CAD build for the part. Positions are in the model's coordinates, mm. Face numbers are marked on the shaded views. A direction names the side the tool comes from. Coordinates: 2 decimals unless noted, no trailing zeros. Loops run counter-clockwise (first coordinate to the right, second up) from the corner with the lowest first, then second, coordinate; pieces in that order, holes last. Notation, with made-up numbers: (-9, 17) - (0, 17) arc R28 cw to (0, 39) - close; hole circle Ø9 at (23, 7). An arc over 180 degrees is marked (long way). Put each result on its own line as item: value.
```python
from build123d import *

# Parameters (mm, degrees)
SKETCH1_R           = 60
BOSS_EXTRUDE1_DEPTH = 20
BOSS_EXTRUDE2_DEPTH = 10
SKETCH6_R           = 20.05
CUT_EXTRUDE1_DEPTH  = 92.787798753
SKETCH8_R           = 6.5
CUT_EXTRUDE3_DEPTH  = 10
SKETCH9_R           = 2.000000002
CUT_EXTRUDE4_DEPTH  = 20
SKETCH10_R          = 3.999999996
CUT_EXTRUDE5_DEPTH  = 4


with BuildPart() as part:
    # Sketch1 → Boss-Extrude1 (new body)
    with BuildSketch(Plane(origin=(0, 0, 0), x_dir=(1, 0, 0), z_dir=(0, 1, 0))):
        with Locations(Location((0, 0, 0), (0, 0, 270))):
            Circle(SKETCH1_R)
    extrude(amount=BOSS_EXTRUDE1_DEPTH)

    # Sketch2 → Boss-Extrude2 (add)
    with BuildSketch(Plane.XY.offset(45)):
        with BuildLine():
            Line((-37.344891303, 20), (-37.344891303, 30))
            ThreePointArc((-37.344891303, 30), (-12.344891303, 55), (12.655108697, 30))
            Line((12.655108697, 30), (12.655108697, 20))
            Line((12.655108697, 20), (-37.344891303, 20))
        make_face()
    extrude(amount=-BOSS_EXTRUDE2_DEPTH)

    # Sketch6 → Cut-Extrude1 (cut, through all)
    with BuildSketch(Plane(origin=(0, 20, 0), x_dir=(1, 0, 0), z_dir=(0, 1, 0))):
        with Locations(Location((0, 0, 0), (0, 0, 270))):
            Circle(SKETCH6_R)
    extrude(amount=-CUT_EXTRUDE1_DEPTH, mode=Mode.SUBTRACT)

    # Sketch8 → Cut-Extrude3 (cut)
    with BuildSketch(Plane.XY.offset(45)):
        with Locations((-12.344891303, 40)):
            Circle(SKETCH8_R)
    extrude(amount=-CUT_EXTRUDE3_DEPTH, mode=Mode.SUBTRACT)

    # Sketch9 → Cut-Extrude4 (cut)
    with BuildSketch(Plane(origin=(0, 20, 0), x_dir=(1, 0, 0), z_dir=(0, 1, 0))):
        with Locations(Location((45.655108698, 23.978394329, 0), (0, 0, 270))):
            Circle(SKETCH9_R)
        with Locations(Location((-32.344891302, 23.978394329, 0), (0, 0, 270))):
            Circle(SKETCH9_R)
    extrude(amount=-CUT_EXTRUDE4_DEPTH, mode=Mode.SUBTRACT)

    # Sketch10 → Cut-Extrude5 (cut)
    with BuildSketch(Plane.XZ):
        with Locations(Location((45.655108698, -23.978394329, 0), (0, 0, 270))):
            Circle(SKETCH10_R)
        with Locations(Location((-32.344891302, -23.978394329, 0), (0, 0, 270))):
            Circle(SKETCH10_R)
    extrude(amount=-CUT_EXTRUDE5_DEPTH, mode=Mode.SUBTRACT)


solid = part.part
```
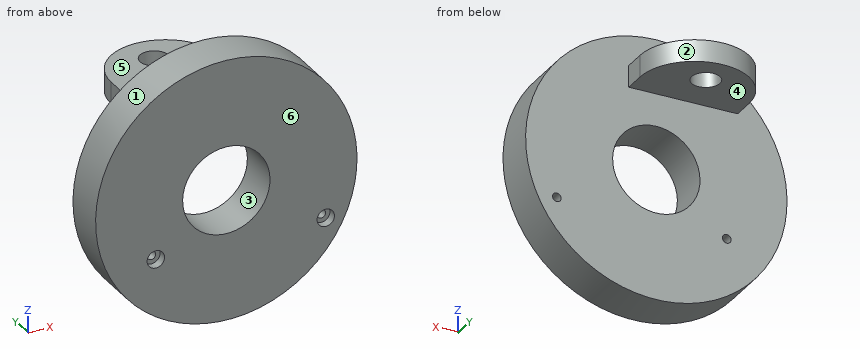
Q1. Tool access for the marked faces 4, 5 and 6: list every direction of +Z, -Z, +X, -X, +Y, -Y with a clear straight run to the whole face (end or side of a thin tool).
Determined:
face 4: -Z, +X, -X, +Y
face 5: +Z, +X, -X, +Y
face 6: +Z, -Z, +X, -X, -Y
Q2. Slice it at B-B, the plane y = 40. Give the cut face in (x, z).
Determined:
outline: (-35.26, 35) - (-18.84, 35) - (-18.84, 45) - (-35.26, 45) - close; (-5.84, 35) - (10.57, 35) - (10.57, 45) - (-5.84, 45) - close
Q3. Pin check, flat tips, straight feed: pin 1 Ø10.5 at (x, y) = (-17.5, 29) entering from -Z; pin 2 Ø2 at (x, z) = (45.5, 8) entering from +Y; pin 3 Ø1.5 at (x, y) = (12.5, 28) entering from +Z. Stop position of each tip, or through.
Determined:
pin 1: z = 35
pin 2: y = 20
pin 3: z = 45
Q4. Slice it at C-C, the plane x = 0. Give the cut face in (y, z), then the cut area to 3 significant figures.
Determined:
outline: (0, -60) - (20, -60) - (20, -20.05) - (0, -20.05) - close; (0, 20.05) - (20, 20.05) - (20, 35) - (51.74, 35) - (51.74, 45) - (20, 45) - (20, 60) - (0, 60) - close
area: 1,920 mm2
Q5. Slice it at D-D, the plane x = 31.5. Give the cut face in (y, z), then the cut area to 3 significant figures.
Determined:
outline: (0, -51.07) - (20, -51.07) - (20, 51.07) - (0, 51.07) - close
area: 2,040 mm2
Q6. Slice it at A-A, the plane z = 0. Give the cut face in (x, y), then the cut area to 3 significant figures.
Determined:
outline: (-60, 0) - (-20.05, 0) - (-20.05, 20) - (-60, 20) - close; (20.05, 0) - (60, 0) - (60, 20) - (20.05, 20) - close
area: 1,600 mm2
Q7. Mould opens along Z. For the marked faces 1, 2 and 3 say: +Z half, -Z half, draft (parallel to the pull), parting line (faces both ways), or undercut.
Determined:
face 1: parting line
face 2: draft
face 3: undercut
Q8. Wall check: L1, parallel to X at y = 15, z = 0; L2, parallel to Y at x = 42.5, z = -24; L3, parallel to Z at x = -12, y = 30. Give the ranges that are in metal, low to high. Write a range as from..to.
Determined:
L1: -60..-20.05, 20.05..60
L2: 4..20
L3: 35..45
